from build123d import *

# Parameters (mm, degrees)
F1_DEPTH = 12.7
F2_R     = 5.08


with BuildPart() as f1:
    # F0 (on Top) → F1 (new body, symmetric)
    with BuildSketch(Plane.XY):
        Polygon((0, 57.169542), (0, 0), (-47.185387, 0), (-47.185387, -45.407388), (45.270618, -45.407388), (45.270618, 57.169542), align=None)
    extrude(amount=F1_DEPTH, both=True)

    # F2
    f2_edges = [f1.edges().sort_by_distance(p)[0] for p in [
        (0, 57.169542, 0),
        (45.270618, 57.169542, 0),
    ]]
    fillet(f2_edges, radius=F2_R)


solid = f1.part
For this review, take the finished solid that the model builds, in its own axes (mm). A direction names the side the tool comes from. Round coordinates to 2 decimals unless told otherwise and drop trailing zeros. Order: outer loops, then holes, each group sorted by start corner. A loop starts at its lowest first (then second) coordinate and runs counter-clockwise, first axis right, second up. Notation, with made-up numbers: M 79,49.5 L 106,49.5 A6 ccw 106,59.5 Z; hole C 52.5,6.25 d5. An arc over 180 degrees is marked long. Use a Markdown table: item, result. Add a question column.
Item 1: Add section C-C, the plane y = 44.5. Give the boundary of the cut face in (x, z).
Item 2: To check wall thickness, follow line 1 along Y through (x, z) = (-38, 3); line 2 along X through (y, z) = (44.5, -7.75); line 3 along Y through (x, z) = (4, -7). State the ranges of each line that lie inside material, in increasing order.
Item 3: Add section B-B, the plane x = -3. Give the boundary of the cut face in (y, z), then the cut area to 3 significant figures.
Item 4: Add section A-A, the plane z = -6. Give the boundary of the cut face in (x, y), then the cut area to 3 significant figures.
Item 5: Tool access review of faces 1 (the flat face through (0, 26, 0)), 2 (the flat face through (-47.185, -22, 0)): name each direction out of +Z, -Z, +X, -X, +Y, -Y from which nothing blocks a thin tool from reaching the whole face with its end or side.
Item 6: Insertion check: pin 1 (7.5 mm diameter, centred on y = 32, z = -2.5, fed in from -X); pin 2 (12.5 mm diameter, centred on x = -20, z = -1.5, fed in from +Y); pin 3 (6 mm diameter, centred on x = 1.5, z = 4.5, fed in from +Y). Each pin has a flat end and moves straight along its axis. Give the tip position at first contact, or say it passes through.
Geometry results:
| question | item | result |
|---|---|---|
| 1 | outline | M 0,-12.7 L 45.27,-12.7 L 45.27,12.7 L 0,12.7 Z |
| 2 | line 1 | y = -45.41 to 0 |
| 2 | line 2 | x = 0 to 45.27 |
| 2 | line 3 | y = -45.41 to 57.05 |
| 3 | outline | M -45.41,-12.7 L 0,-12.7 L 0,12.7 L -45.41,12.7 Z |
| 3 | area | 1,150 mm² |
| 4 | outline | M -47.19,-45.41 L 45.27,-45.41 L 45.27,52.09 A5.08 ccw 40.19,57.17 L 5.08,57.17 A5.08 ccw 0,52.09 L 0,0 L -47.19,0 Z |
| 4 | area | 6,780 mm² |
| 5 | face 1 | +Z, -Z, -X, +Y |
| 5 | face 2 | +Z, -Z, -X, +Y, -Y |
| 6 | pin 1 | stops at x = 0 |
| 6 | pin 2 | stops at y = 0 |
| 6 | pin 3 | stops at y = 57.14 |
